Design review of the part built by this model. Coordinates are the model's own, in mm. Round coordinates to 2 decimals unless told otherwise and drop trailing zeros. Write each loop counter-clockwise with the first axis right and the second up, starting at its lowest first coordinate (ties: lowest second). Pieces come first, ordered by that corner, then holes. Notation, with made-up numbers: M 0.25,37 L 11.25,37 A13 cw 11.25,45 Z; hole C -4,47.5 d4. An arc over 180 degrees is marked long. One line per question, with ' | ' between items. Start each with the question number.
Item 1: For L1, parallel to Y at x = -36.5, z = 0.6; L2, parallel to Y at x = -39, z = 0.5; L3, parallel to X at y = 38, z = 1.1, list the stretches that pass through material, from the lowest coordinate up.
Item 2: Insertion check: pin 1 Ø1 at (x, z) = (-53, 1.5) entering from +Y; pin 2 Ø1 at (x, z) = (-35.5, 2.5) entering from +Y. Each pin has a flat end and moves straight along its axis. Give the tip position at first contact, or say it passes through.
Item 3: Add section C-C, the plane y = 48.5. State the section outline as (x, z) points.
Item 4: Add section A-A, the plane z = 2.5. Give the number of separate pieces and of enclosed holes in the cut face, and give its area (3 significant figures).
Item 5: Draft analysis for pull direction Y (two halves, no side actions). For faces 1 (the face through (-44, -3, 0)), 2 (the face through (-37.21, -46.64, 1.97)), 3 (the face through (-59.922, 24.469, 1.972)), state which applies: released by +Y, released by -Y, zero draft, split by the parting line, or undercut.
Item 6: Add section B-B, the plane y = -44.5. State the section outline as (x, z) points.
```python
from build123d import *

# Parameters (mm, degrees)
F0_R     = 1.425
F1_DEPTH = 4


# Not quite as in the source:
# - a feature names something its author has since deleted; it is built from what else it names


with BuildPart() as f1:
    # F0 (on Top) → F1 (new body)
    with BuildSketch(Plane.XY):
        with BuildLine():
            ThreePointArc((-32.6695806955, 2.2650205107), (-31.9914759382, 11.3900208154), (-29.6618269361, 20.2386473839))
            Line((-29.6618269361, 20.2386473839), (-32.8313113004, 11.5305606615))
            Line((-32.8313113004, 11.5305606615), (-32.6695806955, 2.2650205107))
        make_face()
        with BuildLine():
            Line((-55.2126988023, 11.5305606615), (-58.3821831004, 20.2386472017))
            ThreePointArc((-58.3821831004, 20.2386472017), (-56.126426517, 11.8200489678), (-55.3668141772, 3.1376401385))
            ThreePointArc((-55.3668141772, 3.1376401385), (-55.3687180209, 2.7013137107), (-55.3744294072, 2.2650205107))
            Line((-55.3744294072, 2.2650205107), (-55.2126988023, 11.5305606615))
        make_face()
        with BuildLine():
            Line((-39.6659744052, 56.5204558903), (-48.3780356975, 56.5204558903))
            ThreePointArc((-48.3780356975, 56.5204558903), (-51.6102759902, 55.7295317226), (-54.1121000075, 53.5354909448))
            Line((-54.1121000075, 53.5354909448), (-60.2135254943, 44.8217522976))
            ThreePointArc((-60.2135254943, 44.8217522976), (-61.5591745589, 42.0930459292), (-62.0220050514, 39.0859879341))
            Line((-62.0220050514, 39.0859879341), (-62.0220050514, 36.2389758229))
            Line((-62.0220050514, 36.2389758229), (-48.0220050514, 36.2389758229))
            ThreePointArc((-48.0220050514, 36.2389758229), (-44.0220050514, 40.2389758229), (-40.0220050514, 36.2389758229))
            Line((-40.0220050514, 36.2389758229), (-26.0220050514, 36.2389758229))
            Line((-26.0220050514, 36.2389758229), (-26.0220050514, 39.0859879341))
            ThreePointArc((-26.0220050514, 39.0859879341), (-26.4848355439, 42.0930459292), (-27.8304846085, 44.8217522976))
            Line((-27.8304846085, 44.8217522976), (-33.9319100952, 53.5354909448))
            ThreePointArc((-33.9319100952, 53.5354909448), (-36.4337341126, 55.7295317226), (-39.6659744052, 56.5204558903))
        make_face()
        with BuildLine():
            Line((-49.6788593009, 44.017150416), (-48.6181991291, 42.9564902442))
            ThreePointArc((-48.6181991291, 42.9564902442), (-48.1788593009, 41.8958300724), (-48.6181991291, 40.8351699006))
            ThreePointArc((-48.6181991291, 40.8351699006), (-49.6788593009, 40.3958300724), (-50.7395194726, 40.8351699006))
            Line((-50.7395194726, 40.8351699006), (-51.8001796444, 41.8958300724))
            ThreePointArc((-51.8001796444, 41.8958300724), (-52.2395194726, 42.9564902442), (-51.8001796444, 44.017150416))
            ThreePointArc((-51.8001796444, 44.017150416), (-50.7395194726, 44.4564902442), (-49.6788593009, 44.017150416))
        make_face(mode=Mode.SUBTRACT)
        with BuildLine():
            ThreePointArc((-36.2438304583, 44.017150416), (-35.8044906301, 42.9564902442), (-36.2438304583, 41.8958300724))
            Line((-36.2438304583, 41.8958300724), (-37.3044906301, 40.8351699006))
            ThreePointArc((-37.3044906301, 40.8351699006), (-38.3651508019, 40.3958300724), (-39.4258109737, 40.8351699006))
            ThreePointArc((-39.4258109737, 40.8351699006), (-39.8651508019, 41.8958300724), (-39.4258109737, 42.9564902442))
            Line((-39.4258109737, 42.9564902442), (-38.3651508019, 44.017150416))
            ThreePointArc((-38.3651508019, 44.017150416), (-37.3044906301, 44.4564902442), (-36.2438304583, 44.017150416))
        make_face(mode=Mode.SUBTRACT)
        with BuildLine():
            Line((-31.557524447, -61.4446392968), (-31.8823640322, -42.8345919221))
            ThreePointArc((-31.8823640322, -42.8345919221), (-44.0220050514, -43.7610241771), (-56.1616460705, -42.8345919221))
            Line((-56.1616460705, -42.8345919221), (-56.4864856557, -61.4446392968))
            ThreePointArc((-56.4864856557, -61.4446392968), (-55.9132911637, -62.8813626383), (-54.4867902654, -63.4795441097))
            Line((-54.4867902654, -63.4795441097), (-33.5572198373, -63.4795441097))
            ThreePointArc((-33.5572198373, -63.4795441097), (-32.130718939, -62.8813626383), (-31.557524447, -61.4446392968))
        make_face()
        with Locations((-51.0220050514, -58.0545441097)):
            Circle(F0_R, mode=Mode.SUBTRACT)
        with Locations((-51.0220050514, -48.0545441097)):
            Circle(F0_R, mode=Mode.SUBTRACT)
        with Locations((-44.0220050514, -58.0545441097)):
            Circle(F0_R, mode=Mode.SUBTRACT)
        with Locations((-37.0220050514, -58.0545441097)):
            Circle(F0_R, mode=Mode.SUBTRACT)
        with Locations((-37.0220050514, -48.0545441097)):
            Circle(F0_R, mode=Mode.SUBTRACT)
        with BuildLine():
            Line((-48.0220050514, 36.2389758229), (-62.0220050514, 36.2389758229))
            Line((-62.0220050514, 36.2389758229), (-62.0220050514, 32.00224563))
            ThreePointArc((-62.0220050514, 32.00224563), (-61.8700825815, 30.2657638533), (-61.4189312592, 28.5820441968))
            Line((-61.4189312592, 28.5820441968), (-58.3821831004, 20.2386472017))
            Line((-58.3821831004, 20.2386472017), (-55.2126988023, 11.5305606615))
            Line((-55.2126988023, 11.5305606615), (-55.3744294072, 2.2650205107))
            Line((-55.3744294072, 2.2650205107), (-56.1616460705, -42.8345919221))
            ThreePointArc((-56.1616460705, -42.8345919221), (-44.0220050514, -43.7610241771), (-31.8823640322, -42.8345919221))
            Line((-31.8823640322, -42.8345919221), (-32.6695806955, 2.2650205107))
            Line((-32.6695806955, 2.2650205107), (-32.8313113004, 11.5305606615))
            Line((-32.8313113004, 11.5305606615), (-29.6618269361, 20.2386473839))
            Line((-29.6618269361, 20.2386473839), (-26.6250788435, 28.5820441968))
            ThreePointArc((-26.6250788435, 28.5820441968), (-26.1739275213, 30.2657638533), (-26.0220050514, 32.00224563))
            Line((-26.0220050514, 32.00224563), (-26.0220050514, 36.2389758229))
            Line((-26.0220050514, 36.2389758229), (-40.0220050514, 36.2389758229))
            ThreePointArc((-40.0220050514, 36.2389758229), (-40.3264869213, 34.7082420935), (-41.1935779266, 33.4105486982))
            ThreePointArc((-41.1935779266, 33.4105486982), (-44.0220050514, 32.2389758229), (-46.8504321761, 33.4105486982))
            ThreePointArc((-46.8504321761, 33.4105486982), (-47.7175231814, 34.7082420935), (-48.0220050514, 36.2389758229))
        make_face()
        with Locations((-44.0220050514, -37.0545441097)):
            Circle(F0_R, mode=Mode.SUBTRACT)
        with BuildLine():
            ThreePointArc((-50.7395194726, 31.6427817452), (-49.6788593009, 32.0821215734), (-48.6181991291, 31.6427817452))
            ThreePointArc((-48.6181991291, 31.6427817452), (-48.1788593009, 30.5821215734), (-48.6181991291, 29.5214614017))
            Line((-48.6181991291, 29.5214614017), (-49.6788593009, 28.4608012299))
            ThreePointArc((-49.6788593009, 28.4608012299), (-50.7395194726, 28.0214614017), (-51.8001796444, 28.4608012299))
            ThreePointArc((-51.8001796444, 28.4608012299), (-52.2395194726, 29.5214614017), (-51.8001796444, 30.5821215734))
            Line((-51.8001796444, 30.5821215734), (-50.7395194726, 31.6427817452))
        make_face(mode=Mode.SUBTRACT)
        with BuildLine():
            ThreePointArc((-39.4258109737, 29.5214614017), (-39.8651508019, 30.5821215734), (-39.4258109737, 31.6427817452))
            ThreePointArc((-39.4258109737, 31.6427817452), (-38.3651508019, 32.0821215734), (-37.3044906301, 31.6427817452))
            Line((-37.3044906301, 31.6427817452), (-36.2438304583, 30.5821215734))
            ThreePointArc((-36.2438304583, 30.5821215734), (-35.8044906301, 29.5214614017), (-36.2438304583, 28.4608012299))
            ThreePointArc((-36.2438304583, 28.4608012299), (-37.3044906301, 28.0214614017), (-38.3651508019, 28.4608012299))
            Line((-38.3651508019, 28.4608012299), (-39.4258109737, 29.5214614017))
        make_face(mode=Mode.SUBTRACT)
        with Locations((-51.0220050514, -58.0545441097)):
            Circle(F0_R)
        with Locations((-37.0220050514, -58.0545441097)):
            Circle(F0_R)
    extrude(amount=F1_DEPTH)


solid = f1.part
```
Computed values:
1) L1: y = -63.48 to -49.38, -46.73 to 28.26, 30.84 to 41.64, 44.22 to 55.76 | L2: y = -63.48 to 29.1, 31.94 to 40.54, 43.38 to 56.49 | L3: x = -62.02 to -47.61, -40.43 to -26.02
2) pin 1: stops at y = 55.18 | pin 2: stops at y = 55.48
3) outline: M -57.64,0 L -30.41,0 L -30.41,4 L -57.64,4 Z
4) separate pieces: 1 | enclosed holes: 9 | area: 3,010 mm^2
5) face 1: zero draft | face 2: undercut | face 3: released by -Y
6) outline: M -56.19,0 L -31.85,0 L -31.85,4 L -56.19,4 Z
